Answer from the drawing. Dimensions are ordinates in mm from the lowest x, y and z of the part. A direction names the side the tool comes from. Coordinates: 2 decimals unless noted, no trailing zeros. Order: outer loops, then holes, each group sorted by start corner. A loop starts at its lowest first (then second) coordinate and runs counter-clockwise, first axis right, second up. Notation, with made-up numbers: (58.5, -40) -> (81.5, -40) arc R7 cw to (81.5, -30) -> close; hole circle Ø11 at (-16.75, 36.25). An arc over 180 degrees is marked (long way). Answer in a Markdown table with one row per item.
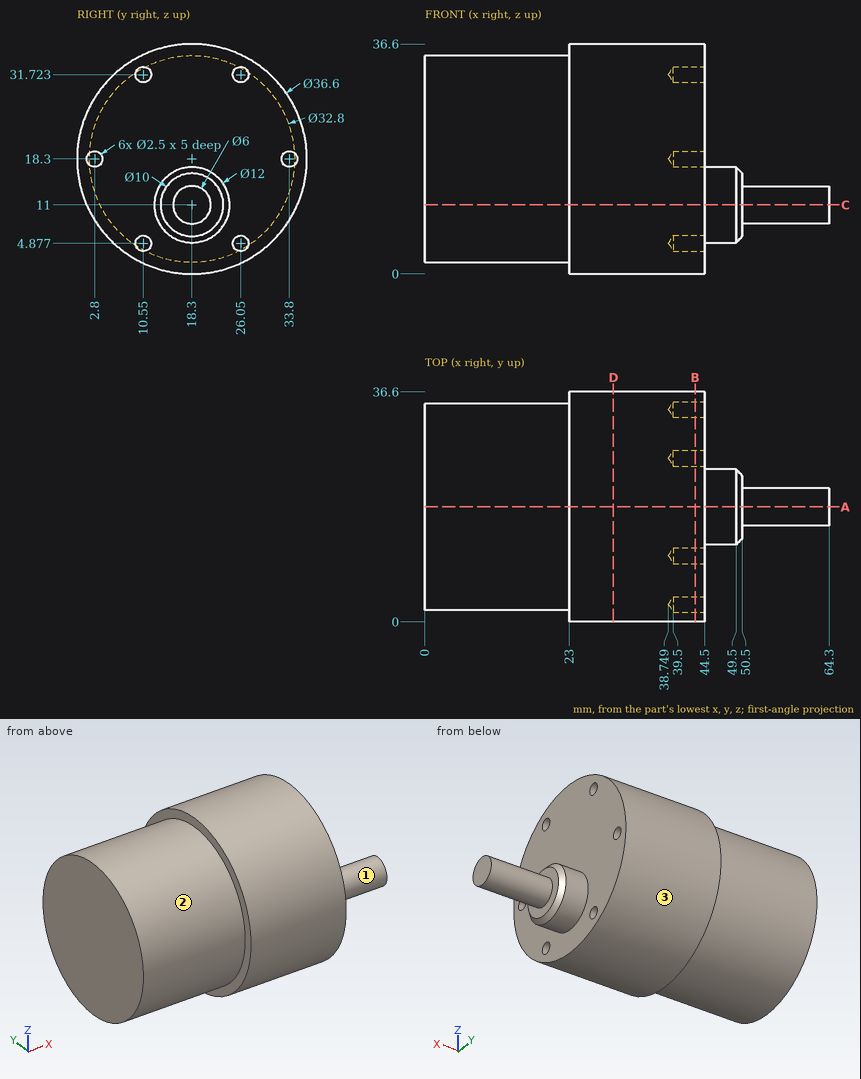
Q1. The part is cut by section A-A (y = 18.3). Write down the section's boundary in (x, z).
Outcome:
| item | result |
|---|---|
| outline | (0, 1.9) -> (23, 1.9) -> (23, 0) -> (44.5, 0) -> (44.5, 5) -> (49.5, 5) -> (50.5, 6) -> (50.5, 8) -> (64.3, 8) -> (64.3, 14) -> (50.5, 14) -> (50.5, 16) -> (49.5, 17) -> (44.5, 17) -> (44.5, 36.6) -> (23, 36.6) -> (23, 34.7) -> (0, 34.7) -> close |
Q2. The part is cut by section D-D (x = 30). Write down the section's boundary in (y, z), then the cut area to 3 significant figures.
Outcome:
| item | result |
|---|---|
| outline | circle Ø36.6 at (18.3, 18.3) |
| area | 1,050 mm² |
Q3. Given pin 1 (3 mm diameter, centred on x = 29, z = 25, fed in from +Y) (1 decimal); pin 2 (1 mm diameter, centred on x = 16.5, y = 28.5, fed in from -Z) (1 decimal); pin 3 (6 mm diameter, centred on x = 46, z = 7, fed in from +Y), each flat-ended and moving along its own axis, determine where each tip first touches the part or whether it passes through.
Outcome:
| item | result |
|---|---|
| pin 1 | y = 35.8 |
| pin 2 | z = 5.1 |
| pin 3 | y = 34.4 |
Q4. The part is cut by section B-B (x = 43). Write down the section's boundary in (y, z).
Outcome:
| item | result |
|---|---|
| outline | circle Ø36.6 at (18.3, 18.3); hole circle Ø2.5 at (2.8, 18.3); hole circle Ø2.5 at (10.55, 4.88); hole circle Ø2.5 at (10.55, 31.72); hole circle Ø2.5 at (26.05, 4.88); hole circle Ø2.5 at (26.05, 31.72); hole circle Ø2.5 at (33.8, 18.3) |
Q5. The part is cut by section C-C (z = 11). Write down the section's boundary in (x, y) (1 decimal), then the cut area to 3 significant figures.
Outcome:
| item | result |
|---|---|
| outline | (0, 3.6) -> (23, 3.6) -> (23, 1.5) -> (44.5, 1.5) -> (44.5, 12.3) -> (49.5, 12.3) -> (50.5, 13.3) -> (50.5, 15.3) -> (64.3, 15.3) -> (64.3, 21.3) -> (50.5, 21.3) -> (50.5, 23.3) -> (49.5, 24.3) -> (44.5, 24.3) -> (44.5, 35.1) -> (23, 35.1) -> (23, 33) -> (0, 33) -> close |
| area | 1,550 mm² |
Q6. Consider line 1 (Z direction, x = 41.5, y = 10) (1 decimal); line 2 (Z direction, x = 43, y = 26) (1 decimal); line 3 (X direction, y = 19.5, z = 20.5). Determine where each line is inside the solid, lowest interval first.
Outcome:
| item | result |
|---|---|
| line 1 | 2 to 3.8, 6 to 30.6, 32.8 to 34.6 |
| line 2 | 1.7 to 3.6, 6.1 to 30.5, 33 to 34.9 |
| line 3 | 0 to 44.5 |
Q7. For the marked faces 1, 2 and 3, determine the directions among +Z, -Z, +X, -X, +Y, -Y from which every point of the face is accessible in a straight line to the end or side of a thin tool.
Outcome:
| item | result |
|---|---|
| face 1 | +X |
| face 2 | -X |
| face 3 | +X, -X |
